Can you work these out from the model? Positions are in its coordinate system, mm. Face numbers are marked on the shaded views. A direction names the side the tool comes from. Give positions to 0.01 mm unless a question says otherwise; leave off trailing zeros. Write each loop counter-clockwise with the first axis right and the second up, starting at its lowest first coordinate (ties: lowest second). Pieces come first, ordered by that corner, then holes. Notation, with made-up numbers: (76.25, 88.25) - (107.25, 88.25) arc R30 ccw to (107.25, 117.25) - close; hole circle Ø5 at (-8.75, 86). An arc over 180 degrees is marked (long way). Return JSON: item names as keys, results as strings. Group by question number.
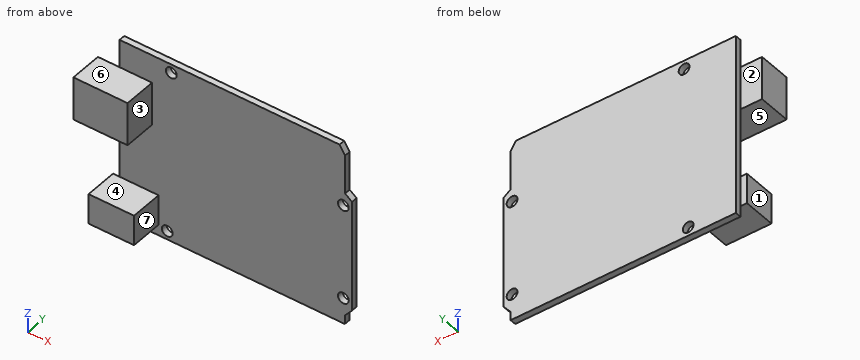
from build123d import *

# Parameters (mm, degrees)
F0_R     = 1.5875
F1_DEPTH = 1.778
F2_W     = 9.525
F2_H     = 12.7
F2_W_2   = 6.35
F3_DEPTH = 9.525
F2_W_3   = 1.905
F2_H_2   = 8.89
F2_W_4   = 11.43
F4_DEPTH = 9.525


with BuildPart() as f1:
    # F0 (on Front) → F1 (new body)
    with BuildSketch(Plane.XZ):
        Polygon((25.218356, 50.8), (-39.297644, 50.8), (-39.297644, -2.54), (26.742356, -2.54), (26.742356, 0), (28.862767, 2.54), (28.862767, 35.306), (26.838946, 36.840845), (26.838946, 48.270845), align=None)
        with Locations((-25.327644, 0)):
            Circle(F0_R, mode=Mode.SUBTRACT)
        with Locations((26.323122, 5.073287)):
            Circle(F0_R, mode=Mode.SUBTRACT)
        with Locations((-24.133679, 48.26)):
            Circle(F0_R, mode=Mode.SUBTRACT)
        with Locations((26.323122, 33.013287)):
            Circle(F0_R, mode=Mode.SUBTRACT)
    extrude(amount=F1_DEPTH)

    # F2 (on face) → F3 (join)
    with BuildSketch(Plane.XZ.offset(1.778)):
        with Locations((-34.535144, 36.195)):
            Rectangle(F2_W, F2_H)
        with Locations((-42.472644, 36.195)):
            Rectangle(F2_W_2, F2_H)
    extrude(amount=F3_DEPTH)

    # F2 (on face) → F4 (join)
    with BuildSketch(Plane.XZ.offset(1.778)):
        with Locations((-40.250144, 5.088352)):
            Rectangle(F2_W_3, F2_H_2)
        with Locations((-33.582644, 5.088352)):
            Rectangle(F2_W_4, F2_H_2)
    extrude(amount=F4_DEPTH)


solid = f1.part
1) We'd pull the mould along Z, two halves only. Please class the marked faces 5, 6 and 7: pulls with the +Z half, pulls with the -Z half, needs draft (parallel to the pull), parting line crosses it, or undercut.
2) On a 3-axis mill with a long thin cutter (end or side, diameter ignored), from which of +Z, -Z, +X, -X, +Y, -Y can I reach the whole of each face in a straight line? I mean the marked faces 1, 2, 3 and 4. Say none if no direction works.
3) I need wall thicknesses on line 1 along Z through (x, y) = (-37.5, -3.25) (3 decimals); line 2 along Y through (x, z) = (2, 0.5); line 3 along X through (y, z) = (-11, 6). Which ranges of each line are inside material? Lowest first, please.
4) Imagine slicing it at C-C, the plane z = 27. Write out the boundary of the cut face in (x, y).
5) Imagine slicing it at A-A, the plane y = -8.25. Write out the boundary of the cut face in (x, z) (3 decimals).
6) Will these pins go through, and if not, where does the flat tip stop? pin 1 Ø3.5 at (x, z) = (26.32, 33.01) entering from -Y; pin 2 Ø3 at (x, z) = (-41, 35.5) entering from +Y; pin 3 Ø0.9 at (y, z) = (-0.5, 43) entering from +X.
7) Imagine slicing it at D-D, the plane x = -20.5. Write out the boundary of the cut face in (y, z), and give its area (3 significant figures).
8) Imagine slicing it at B-B, the plane x = -34.5. Write out the boundary of the cut face in (y, z) (3 decimals).
Resolved:
{
 "1": {"face 5": "undercut", "face 6": "pulls with the +Z half", "face 7": "needs draft"},
 "2": {"face 1": "-Z, -X, +Y, -Y", "face 2": "+Z, -Z, -X, +Y", "face 3": "+Z, +X, -Y", "face 4": "+X, -X, -Y"},
 "3": {"line 1": "0.643 to 9.533, 29.845 to 42.545", "line 2": "-1.78 to 0", "line 3": "-41.2 to -27.87"},
 "4": {"outline": "(-39.3, -1.78) - (28.86, -1.78) - (28.86, 0) - (-39.3, 0) - close"},
 "5": {"outline": "(-45.648, 29.845) - (-29.773, 29.845) - (-29.773, 42.545) - (-45.648, 42.545) - close; (-41.203, 0.643) - (-27.868, 0.643) - (-27.868, 9.533) - (-41.203, 9.533) - close"},
 "6": {"pin 1": "y = -1.78", "pin 2": "y = -1.78", "pin 3": "x = 26.84"},
 "7": {"outline": "(-1.78, -2.54) - (0, -2.54) - (0, 50.8) - (-1.78, 50.8) - close", "area": "94.8 mm^2"},
 "8": {"outline": "(-11.303, 0.643) - (-1.778, 0.643) - (-1.778, -2.54) - (0, -2.54) - (0, 50.8) - (-1.778, 50.8) - (-1.778, 42.545) - (-11.303, 42.545) - (-11.303, 29.845) - (-1.778, 29.845) - (-1.778, 9.533) - (-11.303, 9.533) - close"}
}
